Work out the finished part from the listing and answer in its coordinate system (mm). Coordinates: 2 decimals unless noted, no trailing zeros. Order: outer loops, then holes, each group sorted by start corner. A loop starts at its lowest first (then second) coordinate and runs counter-clockwise, first axis right, second up. Notation, with made-up numbers: M 76,-33.5 L 107,-33.5 A21 ccw 107,-18.5 Z; hole C 77,10 d2. An arc over 180 degrees is marked long. Use a Markdown table: item, result.
Autodesk Inventor part; units mm, degrees
ref_plane "YZ Plane" through (0, 0, 0) normal (1, 0, 0) x (0, 1, 0)
ref_plane "XZ Plane" through (0, 0, 0) normal (0, 1, 0) x (-1, 0, 0)
ref_plane "XY Plane" through (0, 0, 0) normal (0, 0, 1) x (1, 0, 0)
sketch "Sketch1" plane through (0, 0, 0) normal (0, 1, 0) x (-1, 0, 0)
  circle A0 centre (0, 0) radius 20.955
  circle A1 centre (0, 0) radius 4.9606
  circle A2 centre (-17.5514, 0) radius 1.9812
  circle A3 centre (8.7757, -15.2) radius 1.9812
  circle A4 centre (8.7757, 15.2) radius 1.9812
  dimension "d0" = 41.91
  dimension "d1" = 9.9212
  dimension "d2" = 3.9624
  dimension "d5" = 360
extrude "Plate1" add sketch "Sketch1" along normal blind 3.048
equation "\"d7\" = Thickness"
equation "\"BendRadius\" = Thickness"
equation "\"BendReliefWidth\" = Thickness"
equation "\"BendReliefDepth\" = 0.5 * Thickness"
equation "\"CornerReliefSize\" = 4 * Thickness"
equation "\"MinimumRemnant\" = 2 * Thickness"
equation "\"TransitionRadius\" = BendRadius"
equation "\"JacobiRadiusSize\" = BendRadius"
equation "\"GapSize\" = Thickness"
properties part number "disk-sheet-b"
(1) A cutting plane is placed at A-A (x = 0). Determine the outline of the cut face in (y, z) (3 decimals).
Conclusion:
| item | result |
|---|---|
| outline | M 0,-20.955 L 3.048,-20.955 L 3.048,-4.961 L 0,-4.961 Z; M 0,4.961 L 3.048,4.961 L 3.048,20.955 L 0,20.955 Z |
(2) A cutting plane is placed at B-B (z = 0). Determine the outline of the cut face in (x, y) (3 decimals).
Conclusion:
| item | result |
|---|---|
| outline | M -20.955,0 L -4.961,0 L -4.961,3.048 L -20.955,3.048 Z; M 4.961,0 L 15.57,0 L 15.57,3.048 L 4.961,3.048 Z; M 19.533,0 L 20.955,0 L 20.955,3.048 L 19.533,3.048 Z |
(3) A cutting plane is placed at D-D (y = 1.95). Determine the outline of the cut face in (x, z) (3 decimals), then the cut area to 3 significant figures.
Conclusion:
| item | result |
|---|---|
| outline | C 0,0 d41.91; hole C -8.776,-15.2 d3.962; hole C -8.776,15.2 d3.962; hole C 0,0 d9.921; hole C 17.551,0 d3.962 |
| area | 1,270 mm2 |
(4) A cutting plane is placed at C-C (z = 15.2). Determine the outline of the cut face in (x, y), then the cut area to 3 significant figures.
Conclusion:
| item | result |
|---|---|
| outline | M -14.42,0 L -10.76,0 L -10.76,3.05 L -14.42,3.05 Z; M -6.79,0 L 14.42,0 L 14.42,3.05 L -6.79,3.05 Z |
| area | 75.9 mm2 |
(5) Given P1, Ø6.5, axis at x = -8.78, z = -15.2, coming from the -Y side; P2, Ø1.5, axis at x = -15.5, y = 2.5, coming from the +Z side, each flat-ended and moving along its own axis, determine where each tip first touches the part or whether it passes through.
Conclusion:
| item | result |
|---|---|
| P1 | y = 0 |
| P2 | z = 14.88 |
(6) Determine the mould class of faces 1 (the flat face through (-4, 0, -4)), 2 (the cylindrical face through (-8.346, 1.503, 17.134)), 3 (the cylindrical face through (2.728, 1.503, -20.777)) for opening direction X: pulls with the +X half, pulls with the -X half, needs draft (parallel to the pull), parting line crosses it, or undercut.
Conclusion:
| item | result |
|---|---|
| face 1 | needs draft |
| face 2 | undercut |
| face 3 | parting line crosses it |
(7) Straight lines are drawn through the part: L1, parallel to X at y = 2.35, z = -1; L2, parallel to X at y = 2.95, z = -0.5; L3, parallel to Z at x = 0, y = 1.5 (3 decimals). For each, find the intervals that lie inside material, in ascending order.
Conclusion:
| item | result |
|---|---|
| L1 | -20.93 to -4.86, 4.86 to 15.84, 19.26 to 20.93 |
| L2 | -20.95 to -4.94, 4.94 to 15.63, 19.47 to 20.95 |
| L3 | -20.955 to -4.961, 4.961 to 20.955 |
